Part model, mm, in its own coordinate system. Give positions to 0.01 mm unless a question says otherwise; leave off trailing zeros. Write each loop counter-clockwise with the first axis right and the second up, starting at its lowest first coordinate (ties: lowest second). Pieces come first, ordered by that corner, then holes. Notation, with made-up numbers: (2, 27.5) - (57, 27.5) arc R11 cw to (57, 35.5) - close; hole circle Ø8 at (-36.75, 10.5). An arc over 180 degrees is marked (long way). Answer in a Markdown table with one row per item. Add a question column.
1. Band-saw the part on A-A on y = 104.5. Write the cut outline in (x, z).
2. Drop flat-ended pins along their axis: pin 1 Ø1.8 at (x, y) = (2, 61.5) entering from +Z; pin 2 Ø3 at (y, z) = (3, 12) entering from +X; pin 3 Ø0.5 at (x, z) = (5.5, 18) entering from +Y; pin 4 Ø2.5 at (y, z) = (3, 9.375) entering from -X. Give the stop position or say it passes through.
3. Probe line 1 along Z through (x, y) = (3.8, 224) (3 decimals); line 2 along Z through (x, y) = (4.7, 154.5); line 3 along Z through (x, y) = (2.5, 183). List the from-to ranges inside material, lowest first.
4. Band-saw the part on B-B on x = 2.25. State how many separate pieces and enclosed holes the cut face has, plus the area to 3 significant figures.
```python
from build123d import *

# Parameters (mm, degrees)
SKETCH_1_W          = 6
SKETCH_1_H          = 30
EXTRUDE_1_DEPTH     = 227
SKETCH_2_R          = 22.5
EXTRUDE_2_DEPTH     = 6
SKETCH_3_R          = 13
CUT_EXTRUDE_1_DEPTH = 231.154839184
HOLE_WIZARD_M32_D   = 3.4
HOLE_WIZARD_M33_D   = 3.4
EXTRUDE_3_DEPTH     = 6
HOLE_WIZARD_M31_D   = 3.4
SKETCH_14_W         = 45
SKETCH_14_H         = 6
CUT_EXTRUDE_2_DEPTH = 1
CUT_EXTRUDE_3_REACH = 232.155
FILLET_1_R          = 2


with BuildPart() as part:
    # Sketch 1 → Extrude 1 (new body)
    with BuildSketch(Plane(origin=(0, 0, 0), x_dir=(1, 0, 0), z_dir=(0, 1, 0))):
        with Locations((3, -15)):
            Rectangle(SKETCH_1_W, SKETCH_1_H)
    extrude(amount=EXTRUDE_1_DEPTH)

    # Sketch 2 → Extrude 2 (add)
    with BuildSketch(Plane.ZY):
        with Locations((15, 113.5)):
            Circle(SKETCH_2_R)
    extrude(amount=-EXTRUDE_2_DEPTH)

    # Sketch 3 → Cut-Extrude 1 (cut, through all)
    with BuildSketch(Plane.ZY):
        with Locations((15, 113.5)):
            Circle(SKETCH_3_R)
    extrude(amount=-CUT_EXTRUDE_1_DEPTH, mode=Mode.SUBTRACT)

    # Hole Wizard M32 (through all)
    with Locations(Plane(origin=(6, -25.024735225, 7.262908886), x_dir=(0, 0, 1), z_dir=(1, 0, 0))):
        with Locations((7.737091114, -157.774735225), (-11.512908886, -138.524735225), (7.737091114, -119.274735225), (26.987091114, -138.524735225)):
            Hole(HOLE_WIZARD_M32_D / 2)

    # Hole Wizard M33 (through all)
    with Locations(Plane(origin=(6, 0, 0), x_dir=(0, 0, -1), z_dir=(1, 0, 0))):
        with Locations((-26, 154.5), (-4, 154.5), (-4, 72.5), (-26, 72.5)):
            Hole(HOLE_WIZARD_M33_D / 2)

    # Sketch 11 → Extrude 3 (add)
    with BuildSketch(Plane(origin=(6, 0, 0), x_dir=(0, 0, -1), z_dir=(1, 0, 0))):
        Polygon((-37.5, 221), (-30, 208.009618943), (0, 208.009618943), (7.5, 221), (7.5, 227), (-37.5, 227), align=None)
        Polygon((0, 18.990381057), (7.5, 6), (7.5, 0), (-37.5, 0), (-37.5, 6), (-30, 18.990381057), align=None)
    extrude(amount=-EXTRUDE_3_DEPTH)

    # Hole Wizard M31 (through all)
    with Locations(Plane(origin=(6, 0, 0), x_dir=(0, 0, -1), z_dir=(1, 0, 0))):
        with Locations((-31.875, 224), (-20.625, 224), (-9.375, 224), (1.875, 224), (-31.875, 3), (-20.625, 3), (-9.375, 3), (1.875, 3)):
            Hole(HOLE_WIZARD_M31_D / 2)

    # Sketch 14 → Cut-Extrude 2 (cut)
    with BuildSketch(Plane(origin=(6, 0, 0), x_dir=(0, 0, -1), z_dir=(1, 0, 0))):
        with Locations((-15, 224)):
            Rectangle(SKETCH_14_W, SKETCH_14_H)
        with Locations((-15, 3)):
            Rectangle(SKETCH_14_W, SKETCH_14_H)
    extrude(amount=-CUT_EXTRUDE_2_DEPTH, mode=Mode.SUBTRACT)

    # Sketch 15 → Cut-Extrude 3 (cut, up to next)
    with BuildSketch(Plane.ZY, mode=Mode.PRIVATE) as cut_extrude_3_sk1:
        with BuildLine():
            Line((13, 91.089065169), (13, 85.005828051))
            Line((13, 85.005828051), (4, 81.730095943))
            Line((4, 81.730095943), (4, 93.872213574))
            ThreePointArc((4, 93.872213574), (8.352708916, 92.004337153), (13, 91.089065169))
        make_face()
    cut_extrude_3_tool1 = extrude(cut_extrude_3_sk1.sketch, amount=-CUT_EXTRUDE_3_REACH, mode=Mode.PRIVATE) & part.part
    # Sketch 15 → Cut-Extrude 3 (cut, up to next)
    with BuildSketch(Plane.ZY, mode=Mode.PRIVATE) as cut_extrude_3_sk2:
        with BuildLine():
            Line((17, 91.089065169), (17, 85.005828051))
            Line((17, 85.005828051), (26, 81.730095943))
            Line((26, 81.730095943), (26, 93.872213574))
            ThreePointArc((26, 93.872213574), (21.647291084, 92.004337153), (17, 91.089065169))
        make_face()
    cut_extrude_3_tool2 = extrude(cut_extrude_3_sk2.sketch, amount=-CUT_EXTRUDE_3_REACH, mode=Mode.PRIVATE) & part.part
    # Sketch 15 → Cut-Extrude 3 (cut, up to next)
    with BuildSketch(Plane.ZY, mode=Mode.PRIVATE) as cut_extrude_3_sk3:
        Polygon((7.538207724, 78.761187147), (15, 81.47705743), (22.461792276, 78.761187147), (15, 72.5), align=None)
    cut_extrude_3_tool3 = extrude(cut_extrude_3_sk3.sketch, amount=-CUT_EXTRUDE_3_REACH, mode=Mode.PRIVATE) & part.part
    # Sketch 15 → Cut-Extrude 3 (cut, up to next)
    with BuildSketch(Plane.ZY, mode=Mode.PRIVATE) as cut_extrude_3_sk4:
        Polygon((4, 68.5), (26, 68.5), (4, 55.798294078), align=None)
    cut_extrude_3_tool4 = extrude(cut_extrude_3_sk4.sketch, amount=-CUT_EXTRUDE_3_REACH, mode=Mode.PRIVATE) & part.part
    # Sketch 15 → Cut-Extrude 3 (cut, up to next)
    with BuildSketch(Plane.ZY, mode=Mode.PRIVATE) as cut_extrude_3_sk5:
        Polygon((4, 51.179491924), (26, 63.881197846), (26, 38.477786002), align=None)
    cut_extrude_3_tool5 = extrude(cut_extrude_3_sk5.sketch, amount=-CUT_EXTRUDE_3_REACH, mode=Mode.PRIVATE) & part.part
    # Sketch 15 → Cut-Extrude 3 (cut, up to next)
    with BuildSketch(Plane.ZY, mode=Mode.PRIVATE) as cut_extrude_3_sk6:
        Polygon((4, 46.560689771), (26, 33.858983849), (4, 21.157277926), align=None)
    cut_extrude_3_tool6 = extrude(cut_extrude_3_sk6.sketch, amount=-CUT_EXTRUDE_3_REACH, mode=Mode.PRIVATE) & part.part
    # Sketch 15 → Cut-Extrude 3 (cut, up to next)
    with BuildSketch(Plane.ZY, mode=Mode.PRIVATE) as cut_extrude_3_sk7:
        Polygon((4, 11), (4, 16.538475773), (26, 29.240181695), (26, 11), align=None)
    cut_extrude_3_tool7 = extrude(cut_extrude_3_sk7.sketch, amount=-CUT_EXTRUDE_3_REACH, mode=Mode.PRIVATE) & part.part
    # Sketch 15 → Cut-Extrude 3 (cut, up to next)
    with BuildSketch(Plane.ZY, mode=Mode.PRIVATE) as cut_extrude_3_sk8:
        Polygon((4, 171.201705922), (4, 158.5), (26, 158.5), align=None)
    cut_extrude_3_tool8 = extrude(cut_extrude_3_sk8.sketch, amount=-CUT_EXTRUDE_3_REACH, mode=Mode.PRIVATE) & part.part
    # Sketch 15 → Cut-Extrude 3 (cut, up to next)
    with BuildSketch(Plane.ZY, mode=Mode.PRIVATE) as cut_extrude_3_sk9:
        with BuildLine():
            Line((26, 145.269904057), (26, 133.127786426))
            ThreePointArc((26, 133.127786426), (21.647291084, 134.995662847), (17, 135.910934831))
            Line((17, 135.910934831), (17, 141.994171949))
            Line((17, 141.994171949), (26, 145.269904057))
        make_face()
    cut_extrude_3_tool9 = extrude(cut_extrude_3_sk9.sketch, amount=-CUT_EXTRUDE_3_REACH, mode=Mode.PRIVATE) & part.part
    # Sketch 15 → Cut-Extrude 3 (cut, up to next)
    with BuildSketch(Plane.ZY, mode=Mode.PRIVATE) as cut_extrude_3_sk10:
        with BuildLine():
            Line((4, 145.269904057), (4, 133.127786426))
            ThreePointArc((4, 133.127786426), (8.352708916, 134.995662847), (13, 135.910934831))
            Line((13, 135.910934831), (13, 141.994171949))
            Line((13, 141.994171949), (4, 145.269904057))
        make_face()
    cut_extrude_3_tool10 = extrude(cut_extrude_3_sk10.sketch, amount=-CUT_EXTRUDE_3_REACH, mode=Mode.PRIVATE) & part.part
    # Sketch 15 → Cut-Extrude 3 (cut, up to next)
    with BuildSketch(Plane.ZY, mode=Mode.PRIVATE) as cut_extrude_3_sk11:
        Polygon((15, 145.52294257), (22.461792276, 148.238812853), (15, 154.5), (7.538207724, 148.238812853), align=None)
    cut_extrude_3_tool11 = extrude(cut_extrude_3_sk11.sketch, amount=-CUT_EXTRUDE_3_REACH, mode=Mode.PRIVATE) & part.part
    # Sketch 15 → Cut-Extrude 3 (cut, up to next)
    with BuildSketch(Plane.ZY, mode=Mode.PRIVATE) as cut_extrude_3_sk12:
        Polygon((4, 175.820508076), (26, 163.118802154), (26, 188.522213998), align=None)
    cut_extrude_3_tool12 = extrude(cut_extrude_3_sk12.sketch, amount=-CUT_EXTRUDE_3_REACH, mode=Mode.PRIVATE) & part.part
    # Sketch 15 → Cut-Extrude 3 (cut, up to next)
    with BuildSketch(Plane.ZY, mode=Mode.PRIVATE) as cut_extrude_3_sk13:
        Polygon((4, 180.439310229), (26, 193.141016151), (4, 205.842722074), align=None)
    cut_extrude_3_tool13 = extrude(cut_extrude_3_sk13.sketch, amount=-CUT_EXTRUDE_3_REACH, mode=Mode.PRIVATE) & part.part
    # Sketch 15 → Cut-Extrude 3 (cut, up to next)
    with BuildSketch(Plane.ZY, mode=Mode.PRIVATE) as cut_extrude_3_sk14:
        Polygon((4, 216), (4, 210.461524227), (26, 197.759818305), (26, 216), align=None)
    cut_extrude_3_tool14 = extrude(cut_extrude_3_sk14.sketch, amount=-CUT_EXTRUDE_3_REACH, mode=Mode.PRIVATE) & part.part
    add(cut_extrude_3_tool1.solids().sort_by_distance((0, 87.736423, 7.983843))[0], mode=Mode.SUBTRACT)
    add(cut_extrude_3_tool2.solids().sort_by_distance((0, 87.736423, 22.016157))[0], mode=Mode.SUBTRACT)
    add(cut_extrude_3_tool3.solids().sort_by_distance((0, 77.579415, 15))[0], mode=Mode.SUBTRACT)
    add(cut_extrude_3_tool4.solids().sort_by_distance((0, 64.266098, 11.333333))[0], mode=Mode.SUBTRACT)
    add(cut_extrude_3_tool5.solids().sort_by_distance((0, 51.179492, 18.666667))[0], mode=Mode.SUBTRACT)
    add(cut_extrude_3_tool6.solids().sort_by_distance((0, 33.858984, 11.333333))[0], mode=Mode.SUBTRACT)
    add(cut_extrude_3_tool7.solids().sort_by_distance((0, 17.510064, 16.958602))[0], mode=Mode.SUBTRACT)
    add(cut_extrude_3_tool8.solids().sort_by_distance((0, 162.733902, 11.333333))[0], mode=Mode.SUBTRACT)
    add(cut_extrude_3_tool9.solids().sort_by_distance((0, 139.263577, 22.016157))[0], mode=Mode.SUBTRACT)
    add(cut_extrude_3_tool10.solids().sort_by_distance((0, 139.263577, 7.983843))[0], mode=Mode.SUBTRACT)
    add(cut_extrude_3_tool11.solids().sort_by_distance((0, 149.420585, 15))[0], mode=Mode.SUBTRACT)
    add(cut_extrude_3_tool12.solids().sort_by_distance((0, 175.820508, 18.666667))[0], mode=Mode.SUBTRACT)
    add(cut_extrude_3_tool13.solids().sort_by_distance((0, 193.141016, 11.333333))[0], mode=Mode.SUBTRACT)
    add(cut_extrude_3_tool14.solids().sort_by_distance((0, 209.489936, 16.958602))[0], mode=Mode.SUBTRACT)

    # Fillet 1
    fillet_1_edges = [part.edges().sort_by_distance(p)[0] for p in [
        (3, 18.990381057, 30),
        (3, 18.990381057, 0),
        (3, 96.729490169, 0),
        (3, 130.270509831, 0),
        (3, 96.729490169, 30),
        (3, 130.270509831, 30),
        (3, 93.872213574, 4),
        (3, 91.089065169, 13),
        (3, 85.005828051, 13),
        (3, 81.730095943, 4),
        (3, 91.089065169, 17),
        (3, 93.872213574, 26),
        (3, 81.730095943, 26),
        (3, 85.005828051, 17),
        (3, 72.5, 15),
        (3, 78.761187147, 7.538207724),
        (3, 81.47705743, 15),
        (3, 78.761187147, 22.461792276),
        (3, 55.798294078, 4),
        (3, 68.5, 4),
        (3, 68.5, 26),
        (3, 38.477786002, 26),
        (3, 51.179491924, 4),
        (3, 63.881197846, 26),
        (3, 21.157277926, 4),
        (3, 46.560689771, 4),
        (3, 33.858983849, 26),
        (3, 11, 26),
        (3, 11, 4),
        (3, 16.538475773, 4),
        (3, 29.240181695, 26),
        (3, 171.201705922, 4),
        (3, 158.5, 26),
        (3, 158.5, 4),
        (3, 141.994171949, 17),
        (3, 145.269904057, 26),
        (3, 133.127786426, 26),
        (3, 135.910934831, 17),
        (3, 135.910934831, 13),
        (3, 133.127786426, 4),
        (3, 145.269904057, 4),
        (3, 141.994171949, 13),
        (3, 145.52294257, 15),
        (3, 148.238812853, 7.538207724),
        (3, 154.5, 15),
        (3, 148.238812853, 22.461792276),
        (3, 175.820508076, 4),
        (3, 188.522213998, 26),
        (3, 163.118802154, 26),
        (3, 180.439310229, 4),
        (3, 205.842722074, 4),
        (3, 193.141016151, 26),
        (3, 216, 4),
        (3, 216, 26),
        (3, 197.759818305, 26),
        (3, 210.461524227, 4),
        (3, 208.009618943, 0),
        (3, 208.009618943, 30),
    ]]
    fillet(fillet_1_edges, radius=FILLET_1_R)


solid = part.part
```
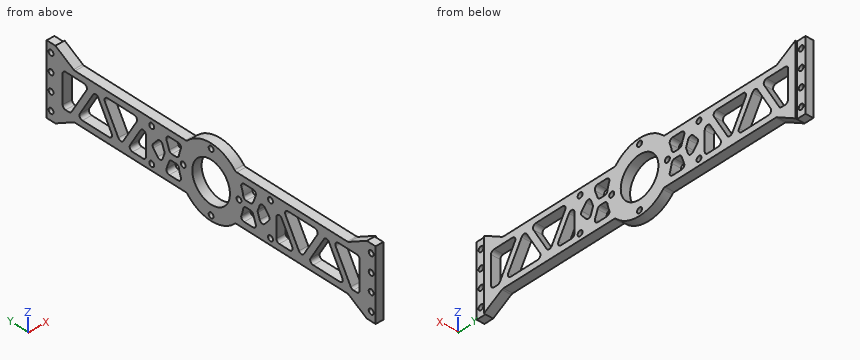
Values:
| question | item | result |
|---|---|---|
| 1 | outline | (0, -5.62) - (6, -5.62) - (6, 5.62) - (0, 5.62) - close; (0, 24.38) - (6, 24.38) - (6, 35.62) - (0, 35.62) - close |
| 2 | pin 1 | stops at z = 30 |
| 2 | pin 2 | stops at x = 5 |
| 2 | pin 3 | stops at y = 221 |
| 2 | pin 4 | passes through |
| 3 | line 1 | z = -7.5 to -3.575, -0.175 to 7.675, 11.075 to 18.925, 22.325 to 30.175, 33.575 to 37.5 |
| 3 | line 2 | z = 0 to 2.3, 5.7 to 24.3, 27.7 to 30 |
| 3 | line 3 | z = 0 to 4.22, 8.44 to 16.44, 26 to 30 |
| 4 | separate pieces | 1 |
| 4 | enclosed holes | 31 |
| 4 | area | 4,590 mm² |
